```python
from build123d import *

# Parameters (mm, degrees)
DOME1_FACE_RADIUS = 0.5
DOME1_HEIGHT      = 0.235
DOME2_FACE_RADIUS = 0.235
DOME2_HEIGHT      = 0.235
FILLET1_R         = 0.25


with BuildPart() as part:
    # Sketch1 → Revolve1 (revolve)
    with BuildSketch(Plane.XY):
        Polygon((0, 0), (0, 3.75), (0.5, 3.75), (0.5, 6.9), (0.675, 6.9), (0.675, 7.4), (0.91, 7.4), (0.91, 6.65), (0.675, 6.65), (0.675, 5.85), (0.765, 5.85), (0.675, 5.51), (0.675, 3.38), (0.545, 3.25), (0.235, 3.25), (0.235, 0), align=None)
    revolve(axis=Axis((0, 0, 0), (0, 1, 0)))

    # Dome1: a dome of height H over a round flat face of radius A is a cap of a sphere of radius (A * A + H * H) / (2 * H)
    dome1_r = (DOME1_FACE_RADIUS * DOME1_FACE_RADIUS + DOME1_HEIGHT * DOME1_HEIGHT) / (2 * DOME1_HEIGHT)
    dome1_base = Plane((0, 3.75, 0), z_dir=(0, 1, 0))
    with Locations(dome1_base.offset(DOME1_HEIGHT - dome1_r)):
        dome1_ball = Sphere(dome1_r, mode=Mode.PRIVATE)
    add(split(dome1_ball, bisect_by=dome1_base, keep=Keep.TOP, mode=Mode.PRIVATE))

    # Dome2: a dome of height H over a round flat face of radius A is a cap of a sphere of radius (A * A + H * H) / (2 * H)
    dome2_r = (DOME2_FACE_RADIUS * DOME2_FACE_RADIUS + DOME2_HEIGHT * DOME2_HEIGHT) / (2 * DOME2_HEIGHT)
    dome2_base = Plane((0, 0, 0), z_dir=(0, -1, 0))
    with Locations(dome2_base.offset(DOME2_HEIGHT - dome2_r)):
        dome2_ball = Sphere(dome2_r, mode=Mode.PRIVATE)
    add(split(dome2_ball, bisect_by=dome2_base, keep=Keep.TOP, mode=Mode.PRIVATE))

    # Fillet1
    fillet1_edges = [part.edges().sort_by_distance(p)[0] for p in [
        (-0.235, 3.25, 0),
    ]]
    fillet(fillet1_edges, radius=FILLET1_R)


solid = part.part
```
Design review of the part built by this model. Coordinates are the model's own, in mm. A direction names the side the tool comes from. Give positions to 0.01 mm unless a question says otherwise; leave off trailing zeros. Write each loop counter-clockwise with the first axis right and the second up, starting at its lowest first coordinate (ties: lowest second). Pieces come first, ordered by that corner, then holes. Notation, with made-up numbers: (36.5, 61) - (91.5, 61) arc R16 ccw to (91.5, 72) - close; hole circle Ø6 at (-18.75, 40.25). An arc over 180 degrees is marked (long way). Return JSON: item names as keys, results as strings. Group by question number.
(1) We need section D-D, the plane y = 7.25. Give the boundary of the cut face in (x, z) (3 decimals).
(2) Insertion check: pin 1 (0.8 mm diameter, centred on x = 0, z = -0.5, fed in from +Y); pin 2 (0.9 mm diameter, centred on x = 0.5, z = 0, fed in from -Y). Each pin has a flat end and moves straight along its axis. Give the tip position at first contact, or say it passes through.
(3) Mouldability with a two-part tool opening along Y and no side actions: class faces 1 (the cylindrical face through (-0.15, 4.43, 0.66)), 2 (the cylindrical face through (-0.15, 6.24, 0.66)) as +Y half, -Y half, draft (parallel to the pull), parting line (faces both ways), or undercut.
(4) Machinability: for faces 3 (the cylindrical face through (-0.108, 5.347, 0.488)), 4 (the cylindrical face through (-0.197, 7.02, 0.888)), which of the approach directions +Z, -Z, +X, -X, +Y, -Y give a long, thin tool a straight path to every point of the face, cutting with its end or side? Answer none if there is none.
(5) To check wall thickness, follow probe 1 along Z at (x, y) = (0, 7.35) (3 decimals); probe 2 along X at (y, z) = (4.25, 0) (3 decimals). State the ranges of each line that lie inside material, in increasing order.
(6) We need section C-C, the plane y = 4.25. Give the boundary of the cut face in (x, z) (3 decimals).
Reported:
{
 "1": {"outline": "circle Ø1.82 at (0, 0); hole circle Ø1.35 at (0, 0)"},
 "2": {"pin 1": "stops at y = 7.4", "pin 2": "stops at y = -0.23"},
 "3": {"face 1": "draft", "face 2": "undercut"},
 "4": {"face 3": "+Y", "face 4": "+Y, -Y"},
 "5": {"probe 1": "z = -0.91 to -0.675, 0.675 to 0.91", "probe 2": "x = -0.675 to -0.5, 0.5 to 0.675"},
 "6": {"outline": "circle Ø1.35 at (0, 0); hole circle Ø1 at (0, 0)"}
}
